from build123d import *

# Parameters (mm, degrees)
CYLINDER_DEPTH                  = 5
CYLINDER_DEPTH_BACK             = 10
SKETCH_1_R                      = 7.5
SKETCH_1_R_2                    = 2.5
SKETCH_2_R                      = 36.75
SKETCH_2_R_2                    = 2.5
BASE_HORIZONT_DEPTH             = 5
SKETCH_3_R                      = 32.75
SKETCH_3_R_2                    = 28.75
EDGE_2_DEPTH                    = 15
SKETCH_4_W                      = 20
SKETCH_4_H                      = 17.5
RECTANGLE_DEPTH                 = 40
RECTANGLE_DIRECTION_2_REACH     = 56.094
SKETCH_6_W                      = 8.2
SKETCH_6_H                      = 17.5
CUT_EXTRUDE_5_DEPTH             = 30
CUT_EXTRUDE_6_REACH             = 76.573
SKETCH_7_R                      = 2.5
CUT_EXTRUDE_7_REACH             = 70.747
SKETCH_8_W                      = 61.662387238
SKETCH_8_H                      = 16.75
CUT_EXTRUDE_7_DIRECTION_2_REACH = 70.747
CUT_EXTRUDE_START               = -40
SKETCH_9_W                      = 20
SKETCH_9_H                      = 5
CUT_EXTRUDE_8_DEPTH             = 40
PIE_REACH                       = 67.583
SKETCH_11_W                     = 5.9
SKETCH_11_H                     = 6.2
EXTRUDE_9_DEPTH                 = 40
FILLET_4_R                      = 6
FILLET_5_R                      = 4


with BuildPart() as part:
    # Эскиз1 → cylinder (new, two sides: drawn at the far end of the back side and taken through both)
    with BuildSketch(Plane(origin=(0, 0, 0), x_dir=(1, 0, 0), z_dir=(0, 1, 0)).offset(-CYLINDER_DEPTH_BACK)):
        with Locations(Location((0, 0, 0), (0, 0, 270))):
            Circle(SKETCH_1_R)
        with Locations(Location((0, 0, 0), (0, 0, 270))):
            Circle(SKETCH_1_R_2, mode=Mode.SUBTRACT)
    extrude(amount=CYLINDER_DEPTH + CYLINDER_DEPTH_BACK)

    # Эскиз2 → base horizont (add)
    with BuildSketch(Plane(origin=(0, 0, 0), x_dir=(1, 0, 0), z_dir=(0, 1, 0))):
        with Locations(Location((0, 0, 0), (0, 0, 270))):
            Circle(SKETCH_2_R)
        with Locations(Location((0, 0, 0), (0, 0, 270))):
            Circle(SKETCH_2_R_2, mode=Mode.SUBTRACT)
    extrude(amount=BASE_HORIZONT_DEPTH)

    # Эскиз3 → edge 2 (add)
    with BuildSketch(Plane(origin=(0, 5, 0), x_dir=(1, 0, 0), z_dir=(0, 1, 0))):
        with Locations(Location((0, 0, 0), (0, 0, 270))):
            Circle(SKETCH_3_R)
        with Locations(Location((0, 0, 0), (0, 0, 270))):
            Circle(SKETCH_3_R_2, mode=Mode.SUBTRACT)
    extrude(amount=-EDGE_2_DEPTH)

    # Эскиз4 → rectangle (add)
    with BuildSketch(Plane(origin=(0, 5, 0), x_dir=(1, 0, 0), z_dir=(0, 1, 0))):
        with Locations((0, 11.25)):
            Rectangle(SKETCH_4_W, SKETCH_4_H)
    extrude(amount=RECTANGLE_DEPTH)

    # rectangle direction 2: up to this face of the body (flat: up to its plane)
    rectangle_direction_2_end = Plane(part.part.faces().sort_by_distance((0, -10, -31.823690117))[0])
    # Эскиз4 → rectangle direction 2 (add, up to the picked face)
    with BuildSketch(Plane(origin=(0, 5, 0), x_dir=(1, 0, 0), z_dir=(0, 1, 0)), mode=Mode.PRIVATE) as rectangle_direction_2_sk1:
        with Locations((0, 11.25)):
            Rectangle(SKETCH_4_W, SKETCH_4_H)
    rectangle_direction_2_tool1 = split(extrude(rectangle_direction_2_sk1.sketch, amount=-RECTANGLE_DIRECTION_2_REACH, mode=Mode.PRIVATE), bisect_by=rectangle_direction_2_end, keep=Keep.BOTH, mode=Mode.PRIVATE)
    add(rectangle_direction_2_tool1.solids().sort_by(Axis((0, 5, -11.25), (0, -1, 0)))[0])

    # Эскиз6 → Вытянуть5 (cut)
    with BuildSketch(Plane(origin=(0, 45, 0), x_dir=(1, 0, 0), z_dir=(0, 1, 0))):
        with Locations((0, 11.25)):
            Rectangle(SKETCH_6_W, SKETCH_6_H)
    extrude(amount=-CUT_EXTRUDE_5_DEPTH, mode=Mode.SUBTRACT)

    # Вытянуть6: up to this face of the body (flat: up to its plane)
    cut_extrude_6_end = Plane(part.part.faces().sort_by_distance((-10, 25, -11.25))[0])
    # Эскиз7 → Вытянуть6 (cut, up to the picked face)
    with BuildSketch(Plane(origin=(10, 0, 0), x_dir=(0, 0, -1), z_dir=(1, 0, 0)), mode=Mode.PRIVATE) as cut_extrude_6_sk1:
        with Locations((13.75, 35)):
            Circle(SKETCH_7_R)
    cut_extrude_6_tool1 = split(extrude(cut_extrude_6_sk1.sketch, amount=-CUT_EXTRUDE_6_REACH, mode=Mode.PRIVATE), bisect_by=cut_extrude_6_end, keep=Keep.BOTH, mode=Mode.PRIVATE)
    add(cut_extrude_6_tool1.solids().sort_by(Axis((10, 35, -13.75), (-1, 0, 0)))[0], mode=Mode.SUBTRACT)

    # Эскиз8 → Вытянуть7 (cut, up to next)
    with BuildSketch(Plane(origin=(0, 0, 0), x_dir=(1, 0, 0), z_dir=(0, 1, 0)), mode=Mode.PRIVATE) as cut_extrude_7_sk1:
        with Locations((0, 28.375)):
            Rectangle(SKETCH_8_W, SKETCH_8_H)
    cut_extrude_7_tool1 = extrude(cut_extrude_7_sk1.sketch, amount=CUT_EXTRUDE_7_REACH, mode=Mode.PRIVATE) & part.part
    add(cut_extrude_7_tool1.solids().sort_by_distance((0, 0, -28.375))[0], mode=Mode.SUBTRACT)

    # Эскиз8 → Вытянуть7 direction 2 (cut, up to next)
    with BuildSketch(Plane(origin=(0, 0, 0), x_dir=(1, 0, 0), z_dir=(0, 1, 0)), mode=Mode.PRIVATE) as cut_extrude_7_direction_2_sk1:
        with Locations((0, 28.375)):
            Rectangle(SKETCH_8_W, SKETCH_8_H)
    cut_extrude_7_direction_2_tool1 = extrude(cut_extrude_7_direction_2_sk1.sketch, amount=-CUT_EXTRUDE_7_DIRECTION_2_REACH, mode=Mode.PRIVATE) & part.part
    add(cut_extrude_7_direction_2_tool1.solids().sort_by_distance((0, 0, -28.375))[0], mode=Mode.SUBTRACT)

    # Эскиз9 → Вытянуть8 (cut)
    with BuildSketch(Plane(origin=(0, 45, 0), x_dir=(1, 0, 0), z_dir=(0, 1, 0)).offset(CUT_EXTRUDE_START)):
        with Locations((0, 5)):
            Rectangle(SKETCH_9_W, SKETCH_9_H)
    extrude(amount=CUT_EXTRUDE_8_DEPTH, mode=Mode.SUBTRACT)

    # Эскиз10 → pie (cut, up to next)
    with BuildSketch(Plane(origin=(0, 5, 0), x_dir=(1, 0, 0), z_dir=(0, 1, 0)), mode=Mode.PRIVATE) as pie_sk1:
        with BuildLine():
            Line((-25.111003564, -14), (25.111003564, -14))
            ThreePointArc((25.111003564, -14), (0, -28.75), (-25.111003564, -14))
        make_face()
    pie_tool1 = extrude(pie_sk1.sketch, amount=-PIE_REACH, mode=Mode.PRIVATE) & part.part
    add(pie_tool1.solids().sort_by_distance((0, 5, 20.052651))[0], mode=Mode.SUBTRACT)

    # Эскиз11 → Вытянуть9 (add)
    with BuildSketch(Plane(origin=(0, 5, 0), x_dir=(1, 0, 0), z_dir=(0, 1, 0))):
        with Locations((-7.05, -10.9)):
            Rectangle(SKETCH_11_W, SKETCH_11_H)
        with Locations((7.05, -10.9)):
            Rectangle(SKETCH_11_W, SKETCH_11_H)
    extrude(amount=EXTRUDE_9_DEPTH)

    # Скругление4
    fillet_4_edges = [part.edges().sort_by_distance(p)[0] for p in [
        (10, 5, -13.75),
        (-10, 5, 10.9),
        (10, 5, 10.9),
        (-10, 5, -13.75),
    ]]
    fillet(fillet_4_edges, radius=FILLET_4_R)

    # Скругление5
    fillet_5_edges = [part.edges().sort_by_distance(p)[0] for p in [
        (-4.1, 5, 10.9),
        (4.1, 5, 10.9),
    ]]
    fillet(fillet_5_edges, radius=FILLET_5_R)


solid = part.part
The listing builds one solid part. Answer for the finished solid, in the listing's coordinates (mm). A direction names the side the tool comes from. Give positions to 0.01 mm unless a question says otherwise; leave off trailing zeros. Write each loop counter-clockwise with the first axis right and the second up, starting at its lowest first coordinate (ties: lowest second). Pieces come first, ordered by that corner, then holes.
Item 1: Section A-A, the plane y = 35 is taken. Write down the section's boundary in (x, z).
Item 2: Flat-ended cylindrical pins translate along their axes: P1, Ø5, axis at y = 24.5, z = 12, coming from the +X side; P2, Ø2, axis at x = 12.5, z = 24.5, coming from the -Y side; P3, Ø4, axis at y = 34, z = -11.5, coming from the -X side; P4, Ø3, axis at x = 14.5, y = 4, coming from the +Z side. Find the tip coordinate at first contact, or state that the pin passes through.
Item 3: Determine the mould class of faces 1 (the flat face through (8, 25, 7.8)), 2 (the flat face through (7, 45, 11)), 3 (the cylindrical face through (-1.021, -4.93, 32.734)) for opening direction Z: released by +Z, released by -Z, zero draft, split by the parting line, or undercut.
Item 4: Section D-D, the plane y = 16 is taken. Write down the section's boundary in (x, z), plus the area to 3 significant figures.
Item 5: Which of the six approach directions +Z, -Z, +X, -X, +Y, -Y give full straight-line access (tool end or side, diameter ignored) to faces 4 (the flat face through (10, 28, 11)), 5 (the flat face through (-4.1, 30, -14)), 6 (the flat face through (-10, 28, -14)), 7 (the cylindrical face through (2.959, 6.203, 10.857)), 8 (the flat face through (10, -5, -11))?
Item 6: Section C-C, the plane z = 0 is taken. Write down the section's boundary in (x, y), plus the area to 4 significant figures.
Item 7: Find the intervals of material crossed by line 1 along X through (y, z) = (-4, 0); line 2 along X through (y, z) = (23.5, -9.5); line 3 along Y through (x, z) = (-6.3, -13.75), in increasing order.
Item 8: Section B-B, the plane x = 9 is taken. Write down the section's boundary in (y, z) (3 decimals), plus the area to 3 significant figures.
Completed:
1. outline: (-10, -20) - (-4.1, -20) - (-4.1, -16.25) - (-10, -16.25) - close; (-10, -11.25) - (-4.1, -11.25) - (-4.1, -7.5) - (-10, -7.5) - close; (-10, 7.8) - (-4.1, 7.8) - (-4.1, 14) - (-10, 14) - close; (4.1, -20) - (10, -20) - (10, -16.25) - (4.1, -16.25) - close; (4.1, -11.25) - (10, -11.25) - (10, -7.5) - (4.1, -7.5) - close; (4.1, 7.8) - (10, 7.8) - (10, 14) - (4.1, 14) - close
2. P1: stops at x = 10
2. P2: passes through
2. P3: stops at x = -10
2. P4: stops at z = 34.37
3. face 1: undercut
3. face 2: zero draft
3. face 3: split by the parting line
4. outline: (-10, -20) - (-4.1, -20) - (-4.1, -7.5) - (-10, -7.5) - close; (-10, 7.8) - (-4.1, 7.8) - (-4.1, 14) - (-10, 14) - close; (4.1, -20) - (10, -20) - (10, -7.5) - (4.1, -7.5) - close; (4.1, 7.8) - (10, 7.8) - (10, 14) - (4.1, 14) - close
4. area: 221 mm2
5. face 4: +Z, -Z, +X, +Y
5. face 5: +Z, -Z, +Y
5. face 6: +Z, -Z, -X, +Y
5. face 7: +Z, +Y
5. face 8: -Z, -Y
6. outline: (-36.75, 0) - (-32.75, 0) - (-32.75, -10) - (-28.75, -10) - (-28.75, 0) - (-7.5, 0) - (-7.5, -10) - (-2.5, -10) - (-2.5, 5) - (-36.75, 5) - close; (2.5, -10) - (7.5, -10) - (7.5, 0) - (28.75, 0) - (28.75, -10) - (32.75, -10) - (32.75, 0) - (36.75, 0) - (36.75, 5) - (2.5, 5) - close
6. area: 522.5 mm2
7. line 1: x = -32.75 to -28.75, -7.5 to -2.5, 2.5 to 7.5, 28.75 to 32.75
7. line 2: x = -10 to -4.1, 4.1 to 10
7. line 3: y = -10 to 32.5, 37.5 to 45
8. outline: (-10, -20) - (45, -20) - (45, -7.5) - (5, -7.5) - (5, 7.8) - (45, 7.8) - (45, 14) - (0, 14) - (0, -2.5) - (-10, -2.5) - close; (-10, 27.305) - (5, 27.305) - (5, 35.631) - (0, 35.631) - (0, 31.489) - (-10, 31.489) - close; hole circle Ø5 at (35, -13.75)
8. area: 1,160 mm2
